Autodesk Inventor part; units mm, degrees
ref_plane "YZ Plane" through (0, 0, 0) normal (1, 0, 0) x (0, 1, 0)
ref_plane "XZ Plane" through (0, 0, 0) normal (0, 1, 0) x (-1, 0, 0)
ref_plane "XY Plane" through (0, 0, 0) normal (0, 0, 1) x (1, 0, 0)
sketch "Sketch2" plane through (0, 0, 0) normal (0, 0, 1) x (1, 0, 0)
  arc A0 (4.746, -3.175) -> (4.746, 3.175) centre (4.746, 0) ccw
  arc A1 (0, 3.175) -> (0, -3.175) centre (0, 0) ccw
  line L0 (0, 3.175) -> (4.746, 3.175)
  line L1 (0, -3.175) -> (4.746, -3.175)
  dimension "d14" = 6.35
  dimension "d15" = 6.35
  dimension "d16" = 0
  dimension "d17" = 0
  dimension "d18" = 4.746
  dimension "d19" = 0
extrude "Extrusion2" add sketch "Sketch2" along normal blind 8.509
sketch "Sketch3" plane through (0, 0, 8.509) normal (0, 0, 1) x (1, 0, 0)
  arc A0 (4.746, -3.175) -> (4.746, 3.175) centre (4.746, 0) ccw
  arc A1 (4.746, -3.175) -> (4.746, 3.175) centre (4.746, 0) ccw
  point P0 (0, 0)
  point P1 (7.921, 0)
  dimension "d22" = 4.746
  dimension "d23" = 0
  dimension "d44" = 3.175
hole "Hole1" at (4.746, 0, 8.509) direction (0, 0, -1) diameter 2.459 depth 3.81 tip angle 118
sketch "Sketch4" plane through (0, 0, 0) normal (0, 0, -1) x (-1, 0, 0)
  point P0 (0, 0)
hole "Hole2" at (0, 0, 0) direction (0, 0, 1) diameter 2.459 depth 3.81 tip angle 118
sketch "Sketch5" plane through (0, 0, 0) normal (0, 0, -1) x (-1, 0, 0)
  arc A0 (-4.746, 3.175) -> (-4.746, -3.175) centre (-4.746, 0) ccw
  arc A1 (0, 3.175) -> (0, -3.175) centre (0, 0) ccw
  line L0 (0, 3.175) -> (-4.746, 3.175)
  arc A2 (0, -3.175) -> (0, 3.175) centre (0, 0) ccw
  line L1 (0, -3.175) -> (-4.746, -3.175)
  dimension "d42" = 4.746
extrude "Extrusion3" cut sketch "Sketch5" against normal blind 3.175 from surface at 0 contours L0 A1 L1 A0
sketch "Sketch11" plane through (0, 0, 8.509) normal (0, 0, 1) x (1, 0, 0)
  arc A0 (0, 3.175) -> (0, -3.175) centre (0, 0) ccw
  arc A1 (4.746, -3.175) -> (4.746, 3.175) centre (4.746, 0) ccw
  arc A2 (4.746, 3.175) -> (4.746, -3.175) centre (4.746, 0) ccw
  line L0 (0, 3.175) -> (4.746, 3.175)
  line L1 (4.746, -3.175) -> (0, -3.175)
sketch "Sketch11 outline for Extrusion5" plane through (0, 0, 8.509) normal (0, 0, 1) x (1, 0, 0)
  arc A0 (4.746, -3.175) -> (4.746, 3.175) centre (4.746, 0) cw
  line L0 (0, -3.175) -> (4.746, -3.175)
  arc A1 (0, 3.175) -> (0, -3.175) centre (0, 0) ccw
  line L1 (4.746, 3.175) -> (0, 3.175)
extrude "Extrusion5" cut sketch "Sketch11 outline for Extrusion5" against normal blind 3.175
properties part number "PC104_EM-113 standoff_4.746"
The listing builds one solid part. Answer for the finished solid, in the listing's coordinates (mm). A direction names the side the tool comes from. Give positions to 0.01 mm unless a question says otherwise; leave off trailing zeros. Order: outer loops, then holes, each group sorted by start corner. A loop starts at its lowest first (then second) coordinate and runs counter-clockwise, first axis right, second up. Notation, with made-up numbers: (72.25, -33) -> (83.25, -33) arc R23 cw to (83.25, -10) -> close; hole circle Ø5 at (72.5, 83). An arc over 180 degrees is marked (long way). Answer as a JSON object with one key per item and string values. Group by question number.
Item 1: Determine the mould class of faces 4 (the flat face through (2, 3.175, 4)), 5 (the conical face through (0.064, 0.204, 4.42)), 6 (the cylindrical face through (-2.8, 1.5, 2)) for opening direction Y: pulls with the +Y half, pulls with the -Y half, needs draft (parallel to the pull), parting line crosses it, or undercut.
Item 2: The part is cut by section C-C on x = 2. Write down the section's boundary in (y, z) (3 decimals).
Item 3: The part is cut by section B-B on y = -1.5. Write down the section's boundary in (x, z) (3 decimals).
Item 4: Flat-ended cylindrical pins translate along their axes: pin 1 (2 mm diameter, centred on x = 3.5, z = 7, fed in from +Y); pin 2 (1.9 mm diameter, centred on x = 1, y = -0.5, fed in from +Z); pin 3 (2 mm diameter, centred on x = 0, y = 0, fed in from +Z); pin 4 (2 mm diameter, centred on x = 4.746, y = 0, fed in from -Z) (3 decimals). Find the tip coordinate at first contact, or state that the pin passes through.
Item 5: Consider L1, parallel to X at y = 0, z = 7.6; L2, parallel to X at y = 0, z = 2.05 (1 decimal). Determine where each line is inside the solid, lowest interval first. Write a range as from..to.
Item 6: A tool of negligible diameter and unlimited length cuts with its end or side. For faces 1 (the cylindrical face through (0.748, -0.976, 1.932)), 2 (the cylindrical face through (7.56, -1.47, 6.4)), 3 (the flat face through (2, -3.175, 4)), from which of +Z, -Z, +X, -X, +Y, -Y can it reach the whole face along a straight path? Write none if from no direction.
Result set:
{
 "1": {"face 4": "pulls with the +Y half", "face 5": "undercut", "face 6": "parting line crosses it"},
 "2": {"outline": "(-3.175, 3.175) -> (-2.466, 3.175) -> (-2.466, 0) -> (2.466, 0) -> (2.466, 3.175) -> (3.175, 3.175) -> (3.175, 5.334) -> (1.594, 5.334) -> (1.594, 8.509) -> (-1.594, 8.509) -> (-1.594, 5.334) -> (-3.175, 5.334) -> close"},
 "3": {"outline": "(-2.798, 0) -> (2.798, 0) -> (2.798, 3.175) -> (7.544, 3.175) -> (7.544, 8.509) -> (1.948, 8.509) -> (1.948, 5.334) -> (-2.798, 5.334) -> close"},
 "4": {"pin 1": "y = 3.17", "pin 2": "z = 8.51", "pin 3": "z = 5.33", "pin 4": "z = 3.175"},
 "5": {"L1": "1.57..3.52, 5.98..7.92", "L2": "-3.2..-1.2, 1.2..3.2"},
 "6": {"face 1": "-Z", "face 2": "+Z", "face 3": "+Z, -Z, +X, -X, -Y"}
}
